Input: part model. Units: mm. Frame: model coordinates. A direction names the side the tool comes from. Coordinates: 2 decimals unless noted, no trailing zeros. Order: outer loops, then holes, each group sorted by start corner. A loop starts at its lowest first (then second) coordinate and runs counter-clockwise, first axis right, second up.
from build123d import *

# Parameters (mm, degrees)
BOSS_EXTRUDE2_DEPTH = 4


with BuildPart() as part:
    # Sketch1 → Boss-Extrude2 (new body)
    with BuildSketch(Plane.XY):
        Polygon((-75, -201), (-10, -201), (-10, -205), (10, -205), (10, -201), (75, -201), (75, -205), (91, -205), (91, -191), (95, -191), (95, -171), (91, -171), (91, -81), (95, -81), (95, -61), (91, -61), (91, 61), (95, 61), (95, 81), (91, 81), (91, 171), (95, 171), (95, 191), (91, 191), (91, 205), (75, 205), (75, 201), (10, 201), (10, 205), (-10, 205), (-10, 201), (-75, 201), (-75, 205), (-91, 205), (-91, 191), (-95, 191), (-95, 171), (-91, 171), (-91, 81), (-95, 81), (-95, 61), (-91, 61), (-91, -61), (-95, -61), (-95, -81), (-91, -81), (-91, -171), (-95, -171), (-95, -191), (-91, -191), (-91, -205), (-75, -205), align=None)
        with BuildLine():
            Line((-17.949055326, 171.697819396), (17.949055326, 171.697819396))
            ThreePointArc((17.949055326, 171.697819396), (32.09119095, 165.83995502), (37.949055326, 151.697819396))
            Line((37.949055326, 151.697819396), (37.949055326, 56.741742537))
            ThreePointArc((37.949055326, 56.741742537), (32.09119095, 42.599606914), (17.949055326, 36.741742537))
            Line((17.949055326, 36.741742537), (-17.949055326, 36.741742537))
            ThreePointArc((-17.949055326, 36.741742537), (-32.09119095, 42.599606914), (-37.949055326, 56.741742537))
            Line((-37.949055326, 56.741742537), (-37.949055326, 151.697819396))
            ThreePointArc((-37.949055326, 151.697819396), (-32.09119095, 165.83995502), (-17.949055326, 171.697819396))
        make_face(mode=Mode.SUBTRACT)
        with BuildLine():
            Line((-17.949055326, -166.180135652), (17.949055326, -166.180135652))
            ThreePointArc((17.949055326, -166.180135652), (32.09119095, -160.322271276), (37.949055326, -146.180135652))
            Line((37.949055326, -146.180135652), (37.949055326, -60))
            ThreePointArc((37.949055326, -60), (32.09119095, -45.857864376), (17.949055326, -40))
            Line((17.949055326, -40), (-17.949055326, -40))
            ThreePointArc((-17.949055326, -40), (-32.09119095, -45.857864376), (-37.949055326, -60))
            Line((-37.949055326, -60), (-37.949055326, -146.180135652))
            ThreePointArc((-37.949055326, -146.180135652), (-32.09119095, -160.322271276), (-17.949055326, -166.180135652))
        make_face(mode=Mode.SUBTRACT)
    extrude(amount=BOSS_EXTRUDE2_DEPTH)


solid = part.part
Item 1: Cut plane A-A on y = -109.5. Return loops of the section in (x, z).
Response values:
outline: (-91, 0) - (-37.95, 0) - (-37.95, 4) - (-91, 4) - close; (37.95, 0) - (91, 0) - (91, 4) - (37.95, 4) - close
Item 2: Cut plane C-C on y = -157. Return loops of the section in (x, z), then the cut area to 3 significant figures.
Response values:
outline: (-91, 0) - (-34.77, 0) - (-34.77, 4) - (-91, 4) - close; (34.77, 0) - (91, 0) - (91, 4) - (34.77, 4) - close
area: 450 mm2
Item 3: Pin query (flat end, axial travel): pin 1 Ø1.5 at (x, z) = (65.5, 1) entering from +Y; pin 2 Ø2 at (x, z) = (51, 0.5) entering from -Y; pin 3 Ø1.2 at (y, z) = (202.5, 2) entering from +X. Return the tip coordinate at first contact, or that it passes through.
Response values:
pin 1: stops at y = 201
pin 2: stops at y = -201
pin 3: stops at x = 91
Item 4: Cut plane D-D on z = 1.05. Count the separate pieces of the cut face and the enclosed holes in it, then the cut area to 3 significant figures.
Response values:
separate pieces: 1
enclosed holes: 2
area: 55,100 mm2
Item 5: Ray query, probe 1 along Y at (x, z) = (-12, 2.15); probe 2 along Y at (x, z) = (-4, 2.65); probe 3 along X at (y, z) = (-144.5, 0.9). Return the intervals inside material, ascending.
Response values:
probe 1: y = -201 to -166.18, -40 to 36.74, 171.7 to 201
probe 2: y = -205 to -166.18, -40 to 36.74, 171.7 to 205
probe 3: x = -91 to -37.95, 37.95 to 91
Item 6: Cut plane B-B on x = 4. Return loops of the section in (y, z), then the cut area to 3 significant figures.
Response values:
outline: (-205, 0) - (-166.18, 0) - (-166.18, 4) - (-205, 4) - close; (-40, 0) - (36.74, 0) - (36.74, 4) - (-40, 4) - close; (171.7, 0) - (205, 0) - (205, 4) - (171.7, 4) - close
area: 595 mm2
Item 7: Draft query along Y for faces 1 (the face through (-31.93, 42.44, 1.97)), 2 (the face through (-1, 3, 4)), 3 (the face through (-32.246, -160.166, 1.972)). Return one class per face: pulls with the +Y half, pulls with the -Y half, needs draft (parallel to the pull), parting line crosses it, or undercut.
Response values:
face 1: undercut
face 2: needs draft
face 3: undercut
Item 8: Access query for faces 4 (the face through (-1, 3, 0)), 5 (the face through (32.246, -46.014, 1.972)). Directions: +Z, -Z, +X, -X, +Y, -Y. A direction counts if a zero-diameter tool reaches every point of the face in a straight line with its end or side. Return the directions, or none.
Response values:
face 4: -Z, +X, -X, +Y, -Y
face 5: +Z, -Z
